The model under review builds one solid part; all positions refer to its coordinate system, in mm. Face numbers are marked on the shaded views. A direction names the side the tool comes from. Coordinates: 2 decimals unless noted, no trailing zeros. Loops run counter-clockwise (first coordinate to the right, second up) from the corner with the lowest first, then second, coordinate; pieces in that order, holes last. Notation, with made-up numbers: (33.5, 70) - (65.5, 70) arc R26 cw to (65.5, 106) - close; hole circle Ø7 at (24, -7.75). An arc over 180 degrees is marked (long way). One line per item, written item: value. Start each with the question number.
1. We need section B-B, the plane y = 20.5. Give the boundary of the cut face in (x, z), then the cut area to 3 significant figures.
2. We need section D-D, the plane x = -19.5. Give the boundary of the cut face in (y, z), then the cut area to 3 significant figures.
3. To check wall thickness, follow line 1 (Z direction, x = -14, y = 8); line 2 (X direction, y = 12.5, z = 114.5) (3 decimals); line 3 (Z direction, x = -31, y = 24). State the ranges of each line that lie inside material, in increasing order.
4. Mouldability with a two-part tool opening along X and no side actions: class the marked faces 1, 2 and 3 as +X half, -X half, draft (parallel to the pull), parting line (faces both ways), or undercut.
5. We need section C-C, the plane z = 46.5. Give the boundary of the cut face in (x, y) (3 decimals), then the cut area to 3 significant figures.
6. Insertion check: P1, Ø4, axis at x = -3, z = 69.5, coming from the +Y side; P2, Ø10, axis at x = 12, z = 73.5, coming from the +Y side; P3, Ø0.8, axis at x = 34.5, y = 24.5, coming from the -Z side. Each pin has a flat end and moves straight along its axis. Give the tip position at first contact, or say it passes through.
7. We need section A-A, the plane y = -3. Give the boundary of the cut face in (x, z).
8. For the marked faces 4 and 5, list the 3-axis set-ups (+Z, -Z, +X, -X, +Y, -Y) from which the entire face can be reached by the end or side of a thin tool; tool diameter is ignored.
from build123d import *

# Parameters (mm, degrees)
RESSALTO_EXTRUS_O2_DEPTH = 120
ESBO_O2_W                = 70
ESBO_O2_H                = 50
RESSALTO_EXTRUS_O3_DEPTH = 5
ESBO_O3_W                = 68
ESBO_O3_H                = 4
CORTE_EXTRUS_O1_DEPTH    = 48
ESBO_O5_R                = 0.4
CORTE_EXTRUS_O4_DEPTH    = 127
ESBO_O6_R                = 0.675
CORTE_EXTRUS_O6_DEPTH    = 30
CORTE_EXTRUS_O7_DEPTH    = 4


with BuildPart() as part:
    # Esboço1 → Ressalto-extrusão2 (new body)
    with BuildSketch(Plane.XY):
        with BuildLine():
            Line((35, -22.5), (-35, -22.5))
            Line((-35, -22.5), (-35, 22.5))
            Line((-35, 22.5), (-0.384609579, 12.609888451))
            ThreePointArc((-0.384609579, 12.609888451), (0.03064267, 12.068183293), (0.42886001, 12.622531431))
            Line((0.42886001, 12.622531431), (35, 22.5))
            Line((35, 22.5), (35, -22.5))
        make_face()
    extrude(amount=RESSALTO_EXTRUS_O2_DEPTH)

    # Esboço2 → Ressalto-extrusão3 (add)
    with BuildSketch(Plane.XY.offset(120)):
        with Locations((0, 2.5)):
            Rectangle(ESBO_O2_W, ESBO_O2_H)
    extrude(amount=RESSALTO_EXTRUS_O3_DEPTH)

    # Esboço3 → Corte-extrusão1 (cut)
    with BuildSketch(Plane(origin=(0, 27.5, 0), x_dir=(1, 0, 0), z_dir=(0, 1, 0))):
        with Locations((0, -122)):
            Rectangle(ESBO_O3_W, ESBO_O3_H)
    extrude(amount=-CORTE_EXTRUS_O1_DEPTH, mode=Mode.SUBTRACT)

    # Esboço5 → Corte-extrusão4 (cut)
    with BuildSketch(Plane(origin=(0, 0, 0), x_dir=(-1, 0, 0), z_dir=(0, 0, -1))):
        with Locations((0, 12.5)):
            Circle(ESBO_O5_R)
    extrude(amount=-CORTE_EXTRUS_O4_DEPTH, mode=Mode.SUBTRACT)

    # Esboço6 → Corte-extrusão6 (cut)
    with BuildSketch(Plane.XY.offset(125)):
        with Locations((0, 12.5)):
            Circle(ESBO_O6_R)
    extrude(amount=-CORTE_EXTRUS_O6_DEPTH, mode=Mode.SUBTRACT)

    # Esboço7 → Corte-extrusão7 (cut)
    with BuildSketch(Plane.XY.offset(125)):
        Polygon((0.675, 12.5), (4, 27.5), (0, 27.5), (-4, 27.5), (-0.675, 12.5), align=None)
    extrude(amount=-CORTE_EXTRUS_O7_DEPTH, mode=Mode.SUBTRACT)


solid = part.part
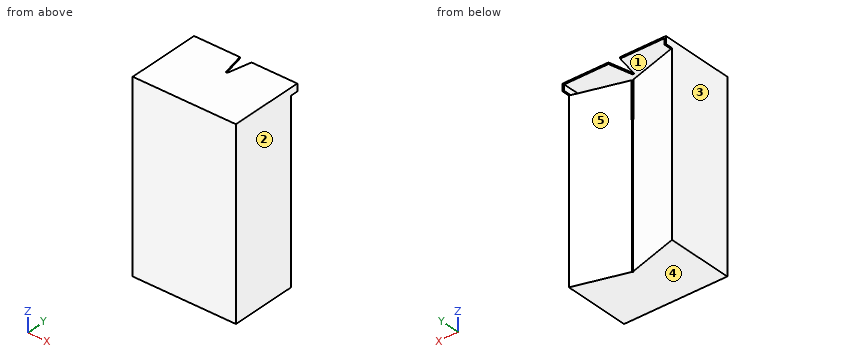
Findings below:
1. outline: (-35, 0) - (-28, 0) - (-28, 120) - (-34, 120) - (-34, 124) - (-2.45, 124) - (-2.45, 125) - (-35, 125) - close; (2.45, 124) - (34, 124) - (34, 120) - (28, 120) - (28, 0) - (35, 0) - (35, 125) - (2.45, 125) - close
1. area: 1,750 mm2
2. outline: (-22.5, 0) - (18.07, 0) - (18.07, 120) - (-20.5, 120) - (-20.5, 124) - (27.5, 124) - (27.5, 125) - (-22.5, 125) - close
2. area: 4,930 mm2
3. line 1: 0 to 120, 124 to 125
3. line 2: -35 to -0.675, 0.675 to 35
3. line 3: 124 to 125
4. face 1: undercut
4. face 2: +X half
4. face 3: -X half
5. outline: (-35, -22.5) - (35, -22.5) - (35, 22.5) - (0.429, 12.623) arc R0.425 cw (long way) to (-0.385, 12.61) - (-35, 22.5) - close
5. area: 2,800 mm2
6. P1: y = 13.93
6. P2: y = 17.36
6. P3: z = 120
7. outline: (-35, 0) - (35, 0) - (35, 125) - (-35, 125) - close; hole (-34, 120) - (34, 120) - (34, 124) - (-34, 124) - close
8. face 4: -Z, +X, -X, +Y, -Y
8. face 5: -Z, +Y
